Could you check a few things on this model? Use its own coordinates, in mm. Face numbers are marked on the shaded views. Round coordinates to 2 decimals unless told otherwise and drop trailing zeros. Loops run counter-clockwise (first coordinate to the right, second up) from the corner with the lowest first, then second, coordinate; pieces in that order, holes last. Notation, with made-up numbers: (49.5, 40.5) -> (70.5, 40.5) arc R19 ccw to (70.5, 73.5) -> close; hole circle Ø9 at (1.5, 43). An arc over 180 degrees is marked (long way). One line per item, written item: value.
from build123d import *

# Parameters (mm, degrees)
SKETCH1_W              = 42
SKETCH1_H              = 126.6
SKETCH1_R              = 1.4732
BASE_FLANGE1_DEPTH     = 1.6002
SKETCHED_BEND1_DEPTH   = 42
SKETCHED_BEND1_2_DEPTH = 42


# Read off the part's stored shape, not the designer's step: Sketched Bend1
# Sheet-metal steps are written as plain solids
with BuildPart() as part:
    # Sketch1 → Base-Flange1 (new body)
    with BuildSketch(Plane(origin=(0, 0, 0), x_dir=(1, 0, 0), z_dir=(0, 1, 0))):
        with Locations((21, -63.3)):
            Rectangle(SKETCH1_W, SKETCH1_H)
        with Locations(Location((6, -16.01, 0), (0, 0, 270))):
            Circle(SKETCH1_R, mode=Mode.SUBTRACT)
        with Locations(Location((36, -16.01, 0), (0, 0, 270))):
            Circle(SKETCH1_R, mode=Mode.SUBTRACT)
    extrude(amount=-BASE_FLANGE1_DEPTH)

    # Sketched Bend1 outline → Sketched Bend1 (cut)
    with BuildSketch(Plane.YZ):
        with BuildLine():
            ThreePointArc((-1.6002, 23.562105466), (-1.172425807, 25.187063933), (0, 26.390765933))
            Line((0, 26.390765933), (0, 126.6))
            Line((0, 126.6), (-1.6002, 126.6))
            Line((-1.6002, 126.6), (-1.6002, 23.562105466))
        make_face()
    extrude(amount=SKETCHED_BEND1_DEPTH, mode=Mode.SUBTRACT)

    # Sketched Bend1 2 outline → Sketched Bend1 2 (add)
    with BuildSketch(Plane.YZ):
        with BuildLine():
            ThreePointArc((0, 23.562105466), (0.497918472, 24.764186994), (1.7, 25.262105466))
            Line((1.7, 25.262105466), (101.062105466, 25.262105466))
            Line((101.062105466, 25.262105466), (101.062105466, 26.862305466))
            Line((101.062105466, 26.862305466), (1.7, 26.862305466))
            ThreePointArc((1.7, 26.862305466), (0.817907384, 26.742236384), (0, 26.390765933))
            Line((0, 26.390765933), (0, 23.562105466))
        make_face()
    extrude(amount=SKETCHED_BEND1_2_DEPTH)


solid = part.part
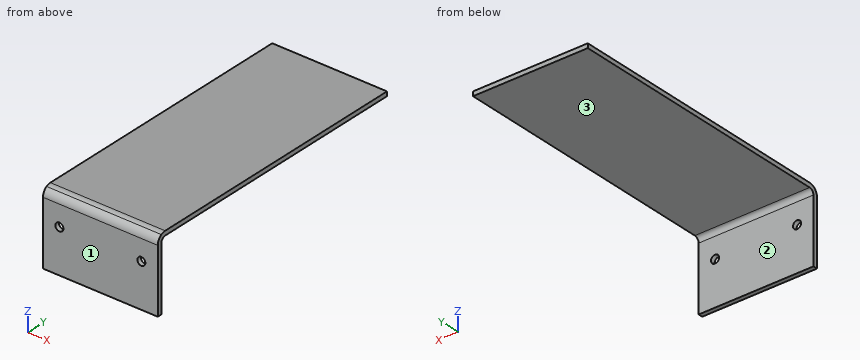
(1) Thinking about a two-plate mould opening in Y: for the marked faces 1, 2 and 3, which applies, released by +Y, released by -Y, zero draft, split by the parting line, or undercut?
Recorded:
face 1: released by -Y
face 2: released by +Y
face 3: zero draft
(2) If I drill on L1, parallel to X at y = -0.65, z = 16.01; L2, parallel to Z at x = 15, y = 93.5; L3, parallel to Y at x = 27.5, z = 8, over which ranges is the centre line in solid material (lowest first)?
Recorded:
L1: 0 to 4.53, 7.47 to 34.53, 37.47 to 42
L2: 25.26 to 26.86
L3: -1.6 to 0
(3) If we section it at C-C, the plane x = 17: Please give me the cut outline in (y, z).
Recorded:
outline: (-1.6, 0) -> (0, 0) -> (0, 23.56) arc R1.7 cw to (1.7, 25.26) -> (101.06, 25.26) -> (101.06, 26.86) -> (1.7, 26.86) arc R3.3 ccw to (-1.6, 23.56) -> close
(4) If we section it at A-A, the plane x = 6: Please give me the cut outline in (y, z).
Recorded:
outline: (-1.6, 0) -> (0, 0) -> (0, 14.54) -> (-1.6, 14.54) -> close; (-1.6, 17.48) -> (0, 17.48) -> (0, 23.56) arc R1.7 cw to (1.7, 25.26) -> (101.06, 25.26) -> (101.06, 26.86) -> (1.7, 26.86) arc R3.3 ccw to (-1.6, 23.56) -> close
(5) If we section it at D-D, the plane y = 63.5: Please give me the cut outline in (x, z), then the cut area to 3 significant figures.
Recorded:
outline: (0, 25.26) -> (42, 25.26) -> (42, 26.86) -> (0, 26.86) -> close
area: 67.2 mm²
(6) I'm going to push a flat-ended pin straight in: pin 1 Ø2.5 at (x, z) = (6, 16.01) entering from +Y. Where does the tip first touch, or does it pass through?
Recorded:
pin 1: through
(7) If we section it at B-B, the plane z = 16.01: Please give me the cut outline in (x, y), then the cut area to 3 significant figures.
Recorded:
outline: (0, -1.6) -> (4.53, -1.6) -> (4.53, 0) -> (0, 0) -> close; (7.47, -1.6) -> (34.53, -1.6) -> (34.53, 0) -> (7.47, 0) -> close; (37.47, -1.6) -> (42, -1.6) -> (42, 0) -> (37.47, 0) -> close
area: 57.8 mm²
